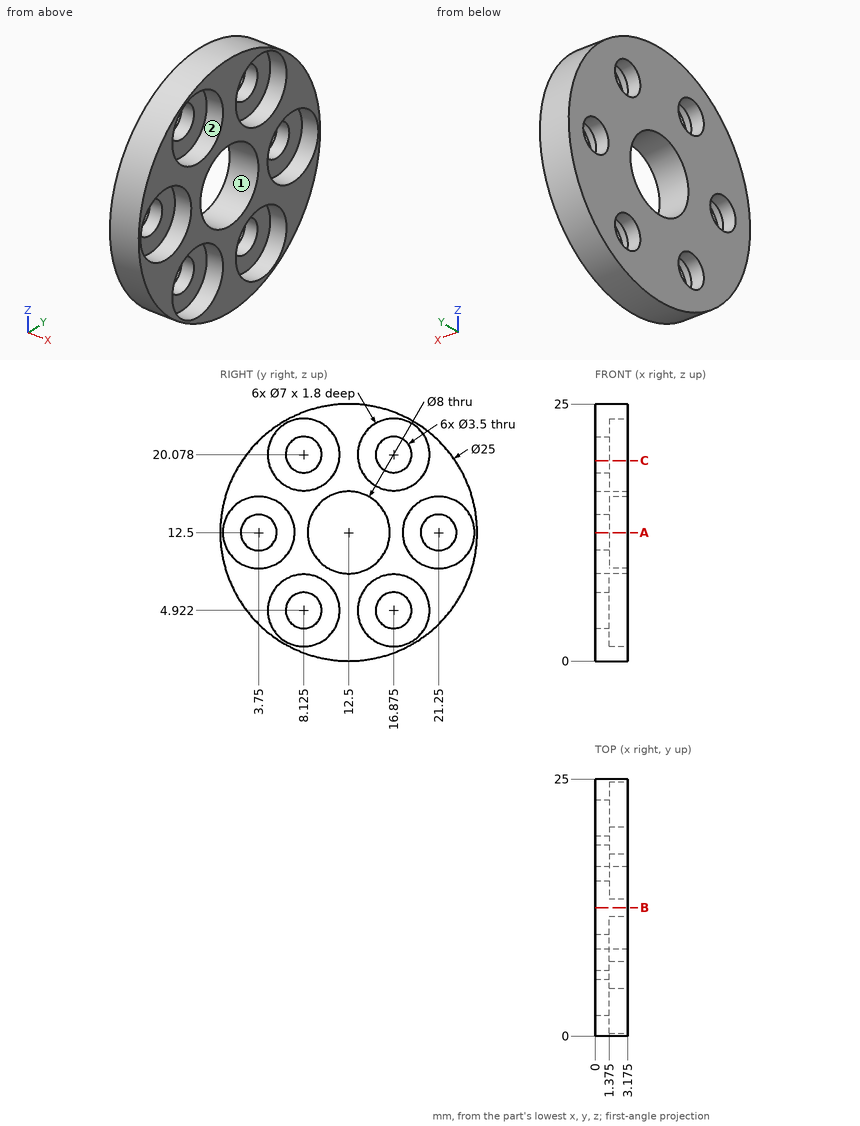
For this review, use the dimensioned drawing (mm, ordinates from the lowest corner) and the shaded views. A direction names the side the tool comes from. Round coordinates to 2 decimals unless told otherwise and drop trailing zeros. Order: outer loops, then holes, each group sorted by start corner. A loop starts at its lowest first (then second) coordinate and runs counter-clockwise, first axis right, second up. Notation, with made-up numbers: (28, -36) -> (34, -36) arc R12 cw to (34, -27) -> close; hole circle Ø4 at (10.25, 46). An arc over 180 degrees is marked (long way). One line per item, written item: value. Start each with the question number.
Q1. Clearance check with flat-ended pins moving along their axes: pin 1 Ø9 at (y, z) = (16.88, 4.92) entering from +X (3 decimals); pin 2 Ø4 at (y, z) = (16.88, 20.08) entering from +X (3 decimals). State where each tip first meets the part, or that it passes through.
Q2. Take a section at B-B (y = 12.5). Write out the cut boundary in (x, z) (1 decimal).
Q3. Machinability: for the marked faces 1 and 2, which of the approach directions +Z, -Z, +X, -X, +Y, -Y give a long, thin tool a straight path to every point of the face, cutting with its end or side? Answer none if there is none.
Q4. Wall thickness on line 1 (Y direction, x = 2, z = 12.5); line 2 (Z direction, x = 2.9, y = 9.25) (1 decimal); line 3 (Z direction, x = 2.8, y = 11.25) (1 decimal): over which ranges is each line inside the solid? List them lowest first.
Q5. Take a section at C-C (z = 19.5). Write out the cut boundary in (x, y) (1 decimal).
Q6. Take a section at A-A (z = 12.5). Count the separate pieces of the cut face and the enclosed holes in it.
Reported:
1. pin 1: stops at x = 3.175
1. pin 2: stops at x = 1.375
2. outline: (0, 0) -> (3.2, 0) -> (3.2, 8.5) -> (0, 8.5) -> close; (0, 16.5) -> (3.2, 16.5) -> (3.2, 25) -> (0, 25) -> close
3. face 1: +X, -X
3. face 2: +X
4. line 1: y = 0 to 0.25, 7.25 to 8.5, 16.5 to 17.75, 24.75 to 25
4. line 2: z = 0.4 to 1.6, 8.2 to 10.2, 14.8 to 16.8, 23.4 to 24.6
4. line 3: z = 0.1 to 3.3, 6.5 to 8.7, 16.3 to 18.5, 21.7 to 24.9
5. outline: (0, 2.1) -> (3.2, 2.1) -> (3.2, 4.7) -> (1.4, 4.7) -> (1.4, 6.5) -> (0, 6.5) -> close; (0, 9.8) -> (1.4, 9.8) -> (1.4, 11.6) -> (3.2, 11.6) -> (3.2, 13.4) -> (1.4, 13.4) -> (1.4, 15.2) -> (0, 15.2) -> close; (0, 18.5) -> (1.4, 18.5) -> (1.4, 20.3) -> (3.2, 20.3) -> (3.2, 22.9) -> (0, 22.9) -> close
6. separate pieces: 4
6. enclosed holes: 0
